Check sheet for the drawn part. Datum: minimum x, y, z corner. Units: mm. A direction names the side the tool comes from. Round coordinates to 2 decimals unless told otherwise and drop trailing zeros. Write each loop counter-clockwise with the first axis right and the second up, starting at its lowest first coordinate (ties: lowest second). Pieces come first, ordered by that corner, then holes. Notation, with made-up numbers: M 73.25,72.25 L 112.25,72.25 A32 cw 112.25,105.25 Z; hole C 27.5,65.25 d7. An arc over 180 degrees is marked long. One line per item, written item: value. Start each with the question number.
1. Section check D-D (z = 5). Record the boundary of the cut face in (x, y).
2. Section check C-C (x = 24). Record the boundary of the cut face in (y, z), and give its area (3 significant figures).
3. Access from +Z, -Z, +X, -X, +Y, -Y to the whole of each face (thin tool, end or side, straight path). Record for the marked faces 4, 5 and 6.
4. Release check for a two-part mould opening along Y. For the marked faces 1, 2 and 3 record: pulls with the +Y half, pulls with the -Y half, needs draft (parallel to the pull), parting line crosses it, or undercut.
5. Depth check by flat-ended pin: P1, Ø1.5, axis at y = 21.5, z = 16.5, coming from the -X side; P2, Ø1, axis at x = 22, z = 3.5, coming from the +Y side; P3, Ø5, axis at x = 16, y = 16, coming from the +Z side; P4, Ø1, axis at y = 28.5, z = 3, coming from the -X side. Enter the tip coordinate at first touch or a pass-through.
6. Section check A-A (y = 16). Record the boundary of the cut face in (x, z), and give its area (3 significant figures).
7. Scan lines: probe 1 along Y at (x, z) = (16, 12.5); probe 2 along Z at (x, y) = (28, 8.5); probe 3 along Y at (x, z) = (16, 5). Record each from-to range of solid material in increasing order. Write a range as [from, to].
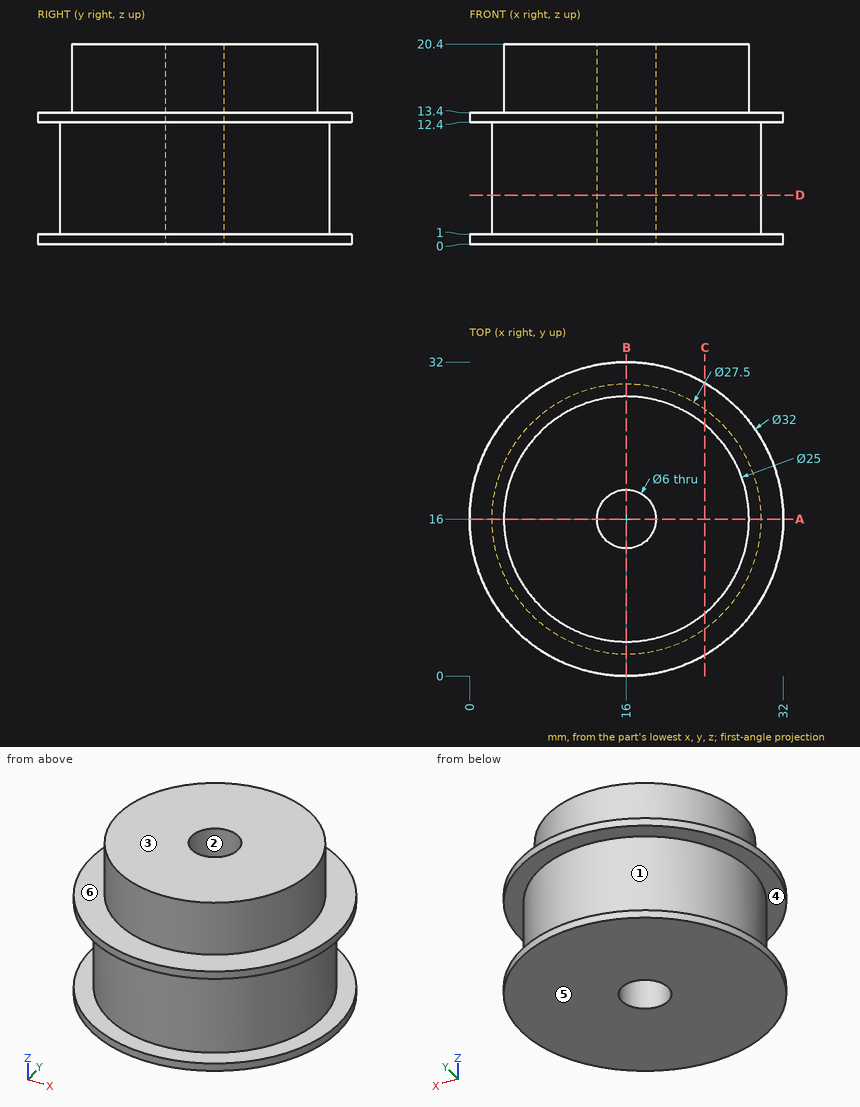
Result sheet:
1. outline: C 16,16 d27.5; hole C 16,16 d6
2. outline: M 2.14,0 L 29.86,0 L 29.86,1 L 27.18,1 L 27.18,12.4 L 29.86,12.4 L 29.86,13.4 L 25.6,13.4 L 25.6,20.4 L 6.4,20.4 L 6.4,13.4 L 2.14,13.4 L 2.14,12.4 L 4.82,12.4 L 4.82,1 L 2.14,1 Z
2. area: 445 mm2
3. face 4: none
3. face 5: -Z, +X, -X, +Y, -Y
3. face 6: +Z
4. face 1: parting line crosses it
4. face 2: undercut
4. face 3: needs draft
5. P1: stops at x = 4.44
5. P2: stops at y = 28.6
5. P3: passes through
5. P4: stops at x = 9.29
6. outline: M 0,0 L 13,0 L 13,20.4 L 3.5,20.4 L 3.5,13.4 L 0,13.4 L 0,12.4 L 2.25,12.4 L 2.25,1 L 0,1 Z; M 19,0 L 32,0 L 32,1 L 29.75,1 L 29.75,12.4 L 32,12.4 L 32,13.4 L 28.5,13.4 L 28.5,20.4 L 19,20.4 Z
6. area: 430 mm2
7. probe 1: y = [0, 13], [19, 32]
7. probe 2: z = [0, 1], [12.4, 13.4]
7. probe 3: y = [2.25, 13], [19, 29.75]
